```python
from build123d import *

# Parameters (mm, degrees)
REVOLVE1_ANGLE           = 50
REVOLVE1_OTHER_WAY_ANGLE = 50
CUT_EXTRUDE1_DEPTH       = 66.325732245
FILLET1_R                = 5


with BuildPart() as part:
    # Sketch1 → Revolve1 (revolve)
    with BuildSketch(Plane.XY):
        Polygon((40, 0), (40, 41), (15, 35), (0, 35), (0, 0), align=None)
    revolve(axis=Axis((0, 0, 0), (1, 0, 0)), revolution_arc=REVOLVE1_ANGLE)

    # Sketch1 → Revolve1 other way (revolve)
    with BuildSketch(Plane.XY):
        Polygon((40, 0), (40, 41), (15, 35), (0, 35), (0, 0), align=None)
    revolve(axis=Axis((0, 0, 0), (-1, 0, 0)), revolution_arc=REVOLVE1_OTHER_WAY_ANGLE)

    # Sketch2 → Cut-Extrude1 (cut, through all)
    with BuildSketch(Plane(origin=(40, 0, 0), x_dir=(0, 0, -1), z_dir=(1, 0, 0))):
        Polygon((5, 55), (5, 25), (-5, 25), (-5, 55), (-52.677102501, 31.854164121), (-43.180890272, -35.505504787), (23.482121539, -41.698119686), (44.635770916, -16.539288183), (46.488696352, -14.335534211), (49.453653338, 39.53478931), align=None)
    extrude(amount=-CUT_EXTRUDE1_DEPTH, mode=Mode.SUBTRACT)

    # Fillet1
    # the kernel refuses this fillet: 5 mm, written as the material it takes off along each edge
    with BuildSketch(Plane(origin=(0, 12.5, 5), x_dir=(1, 0, 0), z_dir=(0, 1, 0)), Plane(origin=(0, 47.141016151, -5), x_dir=(1, 0, 0), z_dir=(0, -1, 0))) as fillet1_piece_1:
        with BuildLine():
            CenterArc((FILLET1_R, FILLET1_R), FILLET1_R, 180, 90)
            Line((0, FILLET1_R), (0, 0))
            Line((0, 0), (FILLET1_R, 0))
        make_face()
    extrude(amount=34.641016151, mode=Mode.SUBTRACT)


solid = part.part
```
CAD build for the part. Positions are in the model's coordinates, mm. A direction names the side the tool comes from. Coordinates: 2 decimals unless noted, no trailing zeros. Loops run counter-clockwise (first coordinate to the right, second up) from the corner with the lowest first, then second, coordinate; pieces in that order, holes last. Notation, with made-up numbers: (-11.5, 47.5) - (-6.5, 47.5) arc R19 ccw to (-6.5, 69.5) - close; hole circle Ø7 at (45.25, 73). An arc over 180 degrees is marked (long way). Return JSON: item names as keys, results as strings.
1. 3-axis set-ups, long thin cutter, end or side, ignore diameter. For faces 1 (the flat face through (23, 31, 5)), 2 (the cylindrical face through (7, 35, 0)): which of +Z, -Z, +X, -X, +Y, -Y reach the whole face in a straight line?
Result:
{"face 1": "+Z, +X, -X, +Y, -Y", "face 2": "-X, +Y"}
2. Band-saw the part on B-B (y = 26). Give the cut face in (x, z), and give its area (3 significant figures).
Result:
{"outline": "(5, -5) - (40, -5) - (40, 5) - (5, 5) arc R5 ccw to start", "area": "389 mm2"}
3. Band-saw the part on A-A (z = 0). Give the cut face in (x, y), and give its area (3 significant figures).
Result:
{"outline": "(0, 25) - (40, 25) - (40, 41) - (15, 35) - (0, 35) - close", "area": "475 mm2"}
4. Probe L1, parallel to Y at x = 14, z = -0.5; L2, parallel to X at y = 26.25, z = -0.5; L3, parallel to X at y = 27.5, z = 3.25. List the from-to ranges inside material, lowest first. Write a range as from..to.
Result:
{"L1": "y = 25..35", "L2": "x = 0.03..40", "L3": "x = 1.2..40"}
5. Band-saw the part on C-C (x = 7). Give the cut face in (y, z).
Result:
{"outline": "(25, -5) - (34.64, -5) arc R35 ccw to (34.64, 5) - (25, 5) - close"}
